Could you check a few things on this model? Use its own coordinates, in mm. Give positions to 0.01 mm unless a question says otherwise; leave off trailing zeros. Loops run counter-clockwise (first coordinate to the right, second up) from the corner with the lowest first, then second, coordinate; pieces in that order, holes last. Notation, with made-up numbers: (11.5, 13.5) - (51.5, 13.5) arc R21 ccw to (51.5, 40.5) - close; hole circle Ø1 at (62.5, 79). An arc over 180 degrees is marked (long way). Use CSV: the item, a comma, the result in double quotes.
from build123d import *

# Parameters (mm, degrees)
SKETCH1_W           = 36
SKETCH1_H           = 27
SKETCH1_R           = 8
BOSS_EXTRUDE1_DEPTH = 12
SKETCH3_R           = 3.1
CUT_EXTRUDE1_DEPTH  = 35.597687784
FILLET1_R           = 2


with BuildPart() as part:
    # Sketch1 → Boss-Extrude1 (new body)
    with BuildSketch(Plane(origin=(0, 0, 0), x_dir=(1, 0, 0), z_dir=(0, 1, 0))):
        with Locations((0, 13.5)):
            Rectangle(SKETCH1_W, SKETCH1_H)
        with Locations(Location((0, 13.5, 0), (0, 0, 270))):
            Circle(SKETCH1_R, mode=Mode.SUBTRACT)
    extrude(amount=BOSS_EXTRUDE1_DEPTH)

    # Sketch3 → Cut-Extrude1 (cut, through all)
    with BuildSketch(Plane(origin=(0, 0, -27), x_dir=(-1, 0, 0), z_dir=(0, 0, -1))):
        with Locations((13, 6)):
            Circle(SKETCH3_R)
        with Locations((-13, 6)):
            Circle(SKETCH3_R)
    extrude(amount=-CUT_EXTRUDE1_DEPTH, mode=Mode.SUBTRACT)

    # Fillet1
    # the kernel refuses this fillet: 2 mm, written as the material it takes off along each edge
    with BuildSketch(Plane(origin=(16, 10, -25), x_dir=(1, 0, 0), z_dir=(0, 1, 0))) as fillet1_piece_1_section:
        Polygon((0, 0), (FILLET1_R, 0), (FILLET1_R, FILLET1_R), (0, FILLET1_R), align=None)
    fillet1_piece_1 = extrude(amount=FILLET1_R, mode=Mode.PRIVATE)
    fillet1_piece_1 = fillet1_piece_1 - Plane(origin=(16, 10, -25), x_dir=(-0.7071067811865476, 0, 0.7071067811865475), z_dir=(0, 1, 0)) * Sphere(FILLET1_R, mode=Mode.PRIVATE)
    add(fillet1_piece_1, mode=Mode.SUBTRACT)
    with BuildSketch(Plane(origin=(-16, 10, -25), x_dir=(0, 1, 0), z_dir=(-1, 0, 0))) as fillet1_piece_2_section:
        Polygon((0, 0), (FILLET1_R, 0), (FILLET1_R, FILLET1_R), (0, FILLET1_R), align=None)
    fillet1_piece_2 = extrude(amount=FILLET1_R, mode=Mode.PRIVATE)
    fillet1_piece_2 = fillet1_piece_2 - Plane(origin=(-16, 10, -25), x_dir=(0, -0.7071067811865475, 0.7071067811865475), z_dir=(-1, 0, 0)) * Sphere(FILLET1_R, mode=Mode.PRIVATE)
    add(fillet1_piece_2, mode=Mode.SUBTRACT)
    with BuildSketch(Plane(origin=(16, 2, -25), x_dir=(1, 0, 0), z_dir=(0, -1, 0))) as fillet1_piece_3_section:
        Polygon((0, 0), (FILLET1_R, 0), (FILLET1_R, -FILLET1_R), (0, -FILLET1_R), align=None)
    fillet1_piece_3 = extrude(amount=FILLET1_R, mode=Mode.PRIVATE)
    fillet1_piece_3 = fillet1_piece_3 - Plane(origin=(16, 2, -25), x_dir=(-0.7071067811865476, 0, 0.7071067811865475), z_dir=(0, -1, 0)) * Sphere(FILLET1_R, mode=Mode.PRIVATE)
    add(fillet1_piece_3, mode=Mode.SUBTRACT)
    with BuildSketch(Plane(origin=(-16, 2, -25), x_dir=(0, -1, 0), z_dir=(-1, 0, 0))) as fillet1_piece_4_section:
        Polygon((0, 0), (FILLET1_R, 0), (FILLET1_R, -FILLET1_R), (0, -FILLET1_R), align=None)
    fillet1_piece_4 = extrude(amount=FILLET1_R, mode=Mode.PRIVATE)
    fillet1_piece_4 = fillet1_piece_4 - Plane(origin=(-16, 2, -25), x_dir=(0, 0.7071067811865475, 0.7071067811865475), z_dir=(-1, 0, 0)) * Sphere(FILLET1_R, mode=Mode.PRIVATE)
    add(fillet1_piece_4, mode=Mode.SUBTRACT)
    with BuildSketch(Plane(origin=(18, 12, 5), x_dir=(-1, 0, 0), z_dir=(0, 0, -1)), Plane(origin=(-18, 0, -25), x_dir=(0, 1, 0), z_dir=(0, 0, 1))) as fillet1_piece_5:
        with BuildLine():
            CenterArc((FILLET1_R, -FILLET1_R), FILLET1_R, 90, 90)
            Line((0, -FILLET1_R), (0, 0))
            Line((0, 0), (FILLET1_R, 0))
        make_face()
    extrude(amount=30, mode=Mode.SUBTRACT)
    with BuildSketch(Plane(origin=(16, 12, -27), x_dir=(0, 0, 1), z_dir=(-1, 0, 0))) as fillet1_piece_6:
        with BuildLine():
            CenterArc((FILLET1_R, -FILLET1_R), FILLET1_R, 90, 90)
            Line((0, -FILLET1_R), (0, 0))
            Line((0, 0), (FILLET1_R, 0))
        make_face()
    extrude(amount=32, mode=Mode.SUBTRACT)
    with BuildSketch(Plane(origin=(-18, 12, -25), x_dir=(0, -1, 0), z_dir=(0, 0, 1)), Plane(origin=(18, 0, 5), x_dir=(-1, 0, 0), z_dir=(0, 0, -1))) as fillet1_piece_7:
        with BuildLine():
            CenterArc((FILLET1_R, FILLET1_R), FILLET1_R, 180, 90)
            Line((0, FILLET1_R), (0, 0))
            Line((0, 0), (FILLET1_R, 0))
        make_face()
    extrude(amount=30, mode=Mode.SUBTRACT)
    with BuildSketch(Plane(origin=(16, 0, -27), x_dir=(0, 0, 1), z_dir=(-1, 0, 0))) as fillet1_piece_8:
        with BuildLine():
            CenterArc((FILLET1_R, FILLET1_R), FILLET1_R, 180, 90)
            Line((0, FILLET1_R), (0, 0))
            Line((0, 0), (FILLET1_R, 0))
        make_face()
    extrude(amount=32, mode=Mode.SUBTRACT)
    with BuildSketch(Plane(origin=(-18, 2, -27), x_dir=(0, 0, 1), z_dir=(0, 1, 0))) as fillet1_piece_9:
        with BuildLine():
            CenterArc((FILLET1_R, FILLET1_R), FILLET1_R, 180, 90)
            Line((0, FILLET1_R), (0, 0))
            Line((0, 0), (FILLET1_R, 0))
        make_face()
    extrude(amount=8, mode=Mode.SUBTRACT)
    with BuildSketch(Plane(origin=(18, 2, -27), x_dir=(0, 0, 1), z_dir=(0, 1, 0))) as fillet1_piece_10:
        with BuildLine():
            CenterArc((FILLET1_R, -FILLET1_R), FILLET1_R, 90, 90)
            Line((0, -FILLET1_R), (0, 0))
            Line((0, 0), (FILLET1_R, 0))
        make_face()
    extrude(amount=8, mode=Mode.SUBTRACT)


solid = part.part
1) Suppose I cut it at C-C (x = 0). Please give me the cut outline in (y, z), plus the area to 3 significant figures.
Answer below:
outline,"(0, -25) arc R2 ccw to (2, -27) - (10, -27) arc R2 ccw to (12, -25) - (12, -21.5) - (0, -21.5) - close; (0, -5.5) - (12, -5.5) - (12, 0) - (0, 0) - close"
area,"130 mm2"
2) Suppose I cut it at A-A (z = -19.75). Please give me the cut outline in (x, y).
Answer below:
outline,"(-18, 2) arc R2 ccw to (-16, 0) - (-4.99, 0) - (-4.99, 12) - (-16, 12) arc R2 ccw to (-18, 10) - close; (4.99, 0) - (16, 0) arc R2 ccw to (18, 2) - (18, 10) arc R2 ccw to (16, 12) - (4.99, 12) - close; hole circle Ø6.2 at (-13, 6); hole circle Ø6.2 at (13, 6)"
3) I need wall thicknesses on line 1 along Y through (x, z) = (13, -19.75); line 2 along X through (y, z) = (7.5, -23.5); line 3 along X through (y, z) = (7, -13.5). Which ranges of each line are inside material? Lowest first, please.
Answer below:
line 1,"y = 0 to 2.9, 9.1 to 12"
line 2,"x = -18 to -15.71, -10.29 to 10.29, 15.71 to 18"
line 3,"x = -18 to -15.93, -10.07 to -8, 8 to 10.07, 15.93 to 18"
4) I'm going to push a flat-ended pin straight in: P1, Ø5, axis at x = 13, y = 6, coming from the +Z side. Where does the tip first touch, or does it pass through?
Answer below:
P1,"passes through"
5) Suppose I cut it at B-B (y = 9.5). Please give me the cut outline in (x, z), plus the area to 3 significant figures.
Answer below:
outline,"(-18, -25) arc R2 ccw to (-16, -27) - (16, -27) arc R2 ccw to (18, -25) - (18, 0) - (-18, 0) - close; hole circle Ø16 at (0, -13.5)"
area,"769 mm2"
6) We'd pull the mould along Z, two halves only. Please class faces 1 (the cylindrical face through (-7.81, 5.92, -15.23)), 2 (the flat face through (0, 6, -27)), 3 (the flat face through (-18, 6, -12)), 4 (the flat face through (0, 6, 0)): +Z half, -Z half, draft (parallel to the pull), parting line (faces both ways), or undercut.
Answer below:
face 1,"undercut"
face 2,"-Z half"
face 3,"draft"
face 4,"+Z half"
7) Suppose I cut it at D-D (z = -23.5). Please give me the cut outline in (x, y), plus the area to 3 significant figures.
Answer below:
outline,"(-18, 2) arc R2 ccw to (-16, 0) - (16, 0) arc R2 ccw to (18, 2) - (18, 10) arc R2 ccw to (16, 12) - (-16, 12) arc R2 ccw to (-18, 10) - close; hole circle Ø6.2 at (-13, 6); hole circle Ø6.2 at (13, 6)"
area,"368 mm2"
